Could you check a few things on this model? Use its own coordinates, in mm. Face numbers are marked on the shaded views. A direction names the side the tool comes from. Round coordinates to 2 decimals unless told otherwise and drop trailing zeros. Write each loop counter-clockwise with the first axis right and the second up, starting at its lowest first coordinate (ties: lowest second). Pieces come first, ordered by that corner, then holes. Notation, with made-up numbers: (73, 88) - (79, 88) arc R19 ccw to (79, 96) - close; hole circle Ø11 at (11, 78.25). An arc over 180 degrees is marked (long way). Put each result on its own line as item: value.
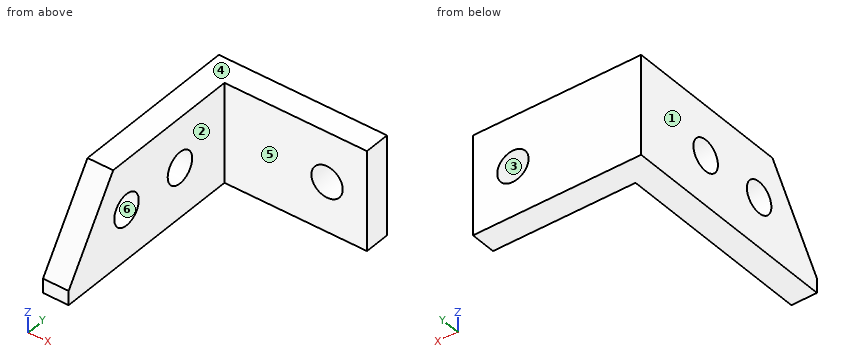
from build123d import *

# Parameters (mm, degrees)
F1_DEPTH = 17.5
F3_D     = 5.5
F4_SIZE2 = 10
F4_SIZE  = 15
F6_D     = 5.5


with BuildPart() as f1:
    # F0 (on Top) → F1 (new body)
    with BuildSketch(Plane.XY):
        Polygon((29.5, 0), (0, 0), (0, -39.5), (4.5, -39.5), (4.5, -4.5), (29.5, -4.5), align=None)
    extrude(amount=F1_DEPTH)

    # F3 (through all)
    with Locations(Plane.XZ.offset(4.5)):
        with Locations((22.5, 8.75)):
            Hole(F3_D / 2)

    # F4
    f4_edges = [f1.edges().sort_by_distance(p)[0] for p in [
        (2.25, -39.5, 17.5),
    ]]
    f4_side = f1.faces().sort_by_distance((2.25, -39.5, 8.75))[0]
    chamfer(f4_edges, length=F4_SIZE, length2=F4_SIZE2, reference=f4_side)

    # F6 (through all)
    with Locations(Plane.YZ.offset(4.5)):
        with Locations((-14.5, 8.75), (-26.5, 8.75)):
            Hole(F6_D / 2)


solid = f1.part
(1) Imagine slicing it at A-A, the plane y = -26.5. List the corners of the cut face in (x, z) for me.
Values found:
outline: (0, 0) - (4.5, 0) - (4.5, 6) - (0, 6) - close; (0, 11.5) - (4.5, 11.5) - (4.5, 17.5) - (0, 17.5) - close
(2) For the marked faces 5 and 6, which set-ups out of +Z, -Z, +X, -X, +Y, -Y let a thin tool reach every point of the face, with its end or its side?
Values found:
face 5: +Z, -Z, +X, -Y
face 6: +X, -X
(3) Please list where these lines run through material, in increasing order: probe 1 along Z at (x, y) = (1.2, -14.5); probe 2 along X at (y, z) = (-10, 12); probe 3 along Y at (x, z) = (9.75, 8). Write a range as from..to.
Values found:
probe 1: z = 0..6, 11.5..17.5
probe 2: x = 0..4.5
probe 3: y = -4.5..0
(4) If we mould it in two halves opening along X, with no side actions, what happens to the marked faces 1, 2, 3 and 4? For each: pulls with the +X half, pulls with the -X half, needs draft (parallel to the pull), parting line crosses it, or undercut.
Values found:
face 1: pulls with the -X half
face 2: pulls with the +X half
face 3: undercut
face 4: needs draft
(5) I'm going to push flat-ended pins straight in: pin 1 (2 mm diameter, centred on x = 13, y = -7, fed in from -Z); pin 2 (9 mm diameter, centred on y = -25, z = 7, fed in from +X); pin 3 (1 mm diameter, centred on x = 3.5, y = -35.5, fed in from +Z); pin 4 (8 mm diameter, centred on x = 25, z = 5.5, fed in from -Y). Where does each tip first touch, or does it pass through?
Values found:
pin 1: passes through
pin 2: stops at x = 4.5
pin 3: stops at z = 9.25
pin 4: stops at y = -4.5
(6) Imagine slicing it at B-B, the plane z = 7.25. List the corners of the cut face in (x, y) for me.
Values found:
outline: (0, -36.33) - (4.5, -36.33) - (4.5, -28.8) - (0, -28.8) - close; (0, -24.2) - (4.5, -24.2) - (4.5, -16.8) - (0, -16.8) - close; (0, -12.2) - (4.5, -12.2) - (4.5, -4.5) - (20.2, -4.5) - (20.2, 0) - (0, 0) - close; (24.8, -4.5) - (29.5, -4.5) - (29.5, 0) - (24.8, 0) - close
(7) Imagine slicing it at D-D, the plane x = 6.5. List the corners of the cut face in (y, z) for me.
Values found:
outline: (-4.5, 0) - (0, 0) - (0, 17.5) - (-4.5, 17.5) - close
(8) Imagine slicing it at C-C, the plane x = 22.5. List the corners of the cut face in (y, z) for me, then the cut area to 3 significant figures.
Values found:
outline: (-4.5, 0) - (0, 0) - (0, 6) - (-4.5, 6) - close; (-4.5, 11.5) - (0, 11.5) - (0, 17.5) - (-4.5, 17.5) - close
area: 54.0 mm^2
